For this review, take the finished solid that the model builds, in its own axes (mm). A direction names the side the tool comes from. Coordinates: 2 decimals unless noted, no trailing zeros. Loops run counter-clockwise (first coordinate to the right, second up) from the corner with the lowest first, then second, coordinate; pieces in that order, holes last. Notation, with made-up numbers: M -11,65.5 L 28,65.5 A21 ccw 28,83.5 Z; hole C 47,69 d9. An arc over 180 degrees is marked long. Answer as a JSON object with one key per item and string values. Group by question number.
Item 1: Add section A-A (y = 0). State the section outline as (x, z) points, then the cut area to 3 significant figures.
Item 2: Tool access review of faces 1 (the face through (-0.29, -2.23, 17.01)), 2 (the face through (0, 0, 35)): name each direction out of +Z, -Z, +X, -X, +Y, -Y from which nothing blocks a thin tool from reaching the whole face with its end or side.
Item 3: Add section B-B (z = 24.5). State the section outline as (x, y) points, then the cut area to 3 significant figures.
Item 4: Wall thickness on L1, parallel to Z at x = -0.75, y = 0; L2, parallel to Z at x = 1.5, y = -1; L3, parallel to X at y = -1, z = 31.5: over which ranges is each line inside the solid? List them lowest first. Write a range as from..to.
Item 5: Mouldability with a two-part tool opening along Y and no side actions: class faces 3 (the face through (1.46, 2.59, -0.06)), 4 (the face through (0, 0, -1)), 5 (the face through (3.031, 0, -1)) as +Y half, -Y half, draft (parallel to the pull), parting line (faces both ways), or undercut.
Item 6: Insertion check: pin 1 (2 mm diameter, centred on x = 0, z = 24, fed in from +Y); pin 2 (3 mm diameter, centred on x = -1.5, z = 7.5, fed in from -Y); pin 3 (1.5 mm diameter, centred on x = 0.5, y = 0, fed in from -Z). Each pin has a flat end and moves straight along its axis. Give the tip position at first contact, or say it passes through.
Autodesk Inventor part; units mm, degrees
ref_plane "YZ Plane" through (0, 0, 0) normal (1, 0, 0) x (0, 1, 0)
ref_plane "XZ Plane" through (0, 0, 0) normal (0, 1, 0) x (-1, 0, 0)
ref_plane "XY Plane" through (0, 0, 0) normal (0, 0, 1) x (1, 0, 0)
sketch "草图1" plane through (0, 0, 0) normal (0, 0, 1) x (1, 0, 0)
  circle A0 centre (0, 0) radius 2.25
  dimension "d0" = 4.5
extrude "拉伸1" add sketch "草图1" along normal blind 35
thread "螺纹1"
sketch "草图4" plane through (0, 0, 0) normal (0, 0, -1) x (-1, 0, 0)
  line L0 (0, -3.5) -> (-3.0311, -1.75)
  line L1 (-3.0311, -1.75) -> (-3.0311, 1.75)
  line L2 (-3.0311, 1.75) -> (0, 3.5)
  line L3 (0, 3.5) -> (3.0311, 1.75)
  line L4 (3.0311, 1.75) -> (3.0311, -1.75)
  line L5 (3.0311, -1.75) -> (0, -3.5)
  point P0 (0, 0)
  point P1 (0, 0)
sketch "草图5" plane through (0, 0, 0) normal (0, 0, -1) x (-1, 0, 0)
  point P0 (0, 0)
extrude "拉伸4" add sketch "草图4" along normal blind 3
fillet "圆角3" radius 0.5 6 edges at (-1.5155, -2.625, -3) (-3.0311, 0, -3) (-1.5155, 2.625, -3) (1.5155, 2.625, -3) (3.0311, 0, -3) (1.5155, -2.625, -3)
fillet "圆角4" radius 0.2 6 edges at (1.5155, -2.625, 0) (3.0311, 0, 0) (1.5155, 2.625, 0) (-1.5155, -2.625, 0) (-1.5155, 2.625, 0) (-3.0311, 0, 0)
sketch "草图6" plane through (0, 0, -3) normal (0, 0, -1) x (-1, 0, 0)
  circle A0 centre (0, 0) radius 1.5
  dimension "d20" = 3
extrude "拉伸5" cut sketch "草图6" against normal blind 2
chamfer "倒角1" distance 0.5 angle 45 1 edges at (-2.25, 0, 35)
equation "\"折弯半径\" = 厚度"
equation "\"折弯释压宽度\" = 厚度"
equation "\"折弯释压深度\" = 0.5 * 厚度"
equation "\"拐角释压尺寸\" = 4 * 厚度"
equation "\"最小余量\" = 2 * 厚度"
equation "\"过渡半径\" = 折弯半径"
equation "\"Jacobi半径尺寸\" = 折弯半径"
equation "\"间隙大小\" = 厚度"
From the geometry:
{
 "1": {"outline": "M -3.03,-2.5 A0.5 ccw -2.53,-3 L -1.5,-3 L -1.5,-1 L 1.5,-1 L 1.5,-3 L 2.53,-3 A0.5 ccw 3.03,-2.5 L 3.03,-0.2 A0.2 ccw 2.83,0 L 2.25,0 L 2.25,34.5 L 1.75,35 L -1.75,35 L -2.25,34.5 L -2.25,0 L -2.83,0 A0.2 ccw -3.03,-0.2 Z", "area": "169 mm²"},
 "2": {"face 1": "+Z", "face 2": "+Z, +X, -X, +Y, -Y"},
 "3": {"outline": "C 0,0 d4.5", "area": "15.9 mm²"},
 "4": {"L1": "z = -1..35", "L2": "z = -3..34.95", "L3": "x = -2.02..2.02"},
 "5": {"face 3": "+Y half", "face 4": "undercut", "face 5": "draft"},
 "6": {"pin 1": "stops at y = 2.25", "pin 2": "stops at y = -2.25", "pin 3": "stops at z = -1"}
}
